Input: part model. Units: mm. Frame: model coordinates. A direction names the side the tool comes from. Give positions to 0.01 mm unless a question says otherwise; leave off trailing zeros. Order: outer loops, then holes, each group sorted by start corner. A loop starts at its lowest first (then second) coordinate and runs counter-clockwise, first axis right, second up. Notation, with made-up numbers: (-31.5, 0.5) - (-15.5, 0.5) arc R32 cw to (-15.5, 35.5) - close; hole circle Ø3 at (7.5, 30). An arc over 180 degrees is marked (long way). Use a Markdown table: item, result.
from build123d import *

# Parameters (mm, degrees)
PAD004_DEPTH            = 7.5
SKETCH007_R             = 1
POCKET002_DEPTH         = 7.001
CHAMFER006_SIZE         = 1
CHAMFER005_SIZE         = 1
BODY003_ROLL_ANGLE      = 180
BODY003_PLACEMENT_ANGLE = 90


with BuildPart() as part:
    # Sketch006 → Pad004 (new body, symmetric)
    with BuildSketch(Plane.XY):
        Polygon((0, 0), (0, -18), (3.25, -18), (3.25, -33.5), (0, -33.5), (0, -41.5), (7, -41.5), (7, 7), align=None)
    extrude(amount=PAD004_DEPTH, both=True)

    # Sketch007 (on Face7 of Pad004) → Pocket002 (cut, through all)
    with BuildSketch(Plane.YZ.offset(7)):
        with Locations((-36.5, 0)):
            Circle(SKETCH007_R)
        with Locations((-15, 0)):
            Circle(SKETCH007_R)
    extrude(amount=-POCKET002_DEPTH, mode=Mode.SUBTRACT)

    # Chamfer006
    chamfer006_edges = [part.edges().sort_by_distance(p)[0] for p in [
        (7, -37.5, 0),
        (7, -16, 0),
    ]]
    chamfer(chamfer006_edges, length=CHAMFER006_SIZE)

    # Chamfer005
    chamfer005_edges = [part.edges().sort_by_distance(p)[0] for p in [
        (7, -17.25, 7.5),
        (7, -41.5, 0),
        (7, -17.25, -7.5),
    ]]
    chamfer(chamfer005_edges, length=CHAMFER005_SIZE)


with BuildPart() as part_1:
    # Body003 roll: moved
    add(part.part.rotate(Axis((0, 0, 0), (1, 0, 0)), BODY003_ROLL_ANGLE))


with BuildPart() as part_2:
    # Body003 placement: moved
    add(part_1.part.rotate(Axis((0, 0, 0), (0, 0, 1)), BODY003_PLACEMENT_ANGLE))


solid = part_2.part
1. Section query C-C (z = 0). Return loops of the section in (x, y), then the cut area to 3 significant figures.
Response:
| item | result |
|---|---|
| outline | (-41.5, 0) - (-37.5, 0) - (-37.5, 6) - (-38.5, 7) - (-40.5, 7) - (-41.5, 6) - close; (-35.5, 0) - (-33.5, 0) - (-33.5, 3.25) - (-18, 3.25) - (-18, 0) - (-16, 0) - (-16, 6) - (-17, 7) - (-34.5, 7) - (-35.5, 6) - close; (-14, 0) - (0, 0) - (7, 7) - (-13, 7) - (-14, 6) - close |
| area | 234 mm^2 |
2. Section query D-D (z = 2.5). Return loops of the section in (x, y), then the cut area to 3 significant figures.
Response:
| item | result |
|---|---|
| outline | (-41.5, 0) - (-33.5, 0) - (-33.5, 3.25) - (-18, 3.25) - (-18, 0) - (0, 0) - (7, 7) - (-40.5, 7) - (-41.5, 6) - close |
| area | 264 mm^2 |
3. Set-up query: faces 1 (the face through (-26, 3.25, 0)), 2 (the face through (-9, 0, 0)). Return all of +Z, -Z, +X, -X, +Y, -Y with unobstructed straight access to the full face (end or side cutting, diameter ignored); none if empty.
Response:
| item | result |
|---|---|
| face 1 | +Z, -Z, -Y |
| face 2 | +Z, -Z, +X, -X, -Y |
4. Section query A-A (x = -15). Return loops of the section in (y, z).
Response:
| item | result |
|---|---|
| outline | (0, -7.5) - (6, -7.5) - (7, -6.5) - (7, -2) - (6, -1) - (0, -1) - close; (0, 1) - (6, 1) - (7, 2) - (7, 6.5) - (6, 7.5) - (0, 7.5) - close |
5. Material intervals for line 1 along X through (y, z) = (3.5, 0); line 2 along X through (y, z) = (5.25, 0.5); line 3 along Z through (x, y) = (-36.5, 3.25), sorted ascending.
Response:
| item | result |
|---|---|
| line 1 | x = -41.5 to -37.5, -35.5 to -16, -14 to 3.5 |
| line 2 | x = -41.5 to -37.37, -35.63 to -15.87, -14.13 to 5.25 |
| line 3 | z = -7.5 to -1, 1 to 7.5 |
6. Pin query (flat end, axial travel): pin 1 (1.8 mm diameter, centred on x = -15, z = 0, fed in from -Y); pin 2 (2.5 mm diameter, centred on y = 1, z = -3.5, fed in from +X); pin 3 (7.5 mm diameter, centred on x = -29, z = -1, fed in from -Y). Return the tip coordinate at first contact, or that it passes through.
Response:
| item | result |
|---|---|
| pin 1 | passes through |
| pin 2 | stops at x = 2.25 |
| pin 3 | stops at y = 3.25 |
7. Mould query, pull axis X, two halves, no side actions, for faces 3 (the face through (-14, 3, 0)), 4 (the face through (-17, 4, 7.5)), 5 (the face through (-41.5, 3, 0)). Classes: pulls with the +X half, pulls with the -X half, needs draft (parallel to the pull), parting line crosses it, or undercut.
Response:
| item | result |
|---|---|
| face 3 | undercut |
| face 4 | needs draft |
| face 5 | pulls with the -X half |
8. Section query B-B (y = 1). Return loops of the section in (x, z), then the cut area to 3 significant figures.
Response:
| item | result |
|---|---|
| outline | (-41.5, -7.5) - (-33.5, -7.5) - (-33.5, 7.5) - (-41.5, 7.5) - close; (-18, -7.5) - (1, -7.5) - (1, 7.5) - (-18, 7.5) - close; hole circle Ø2 at (-36.5, 0); hole circle Ø2 at (-15, 0) |
| area | 399 mm^2 |
